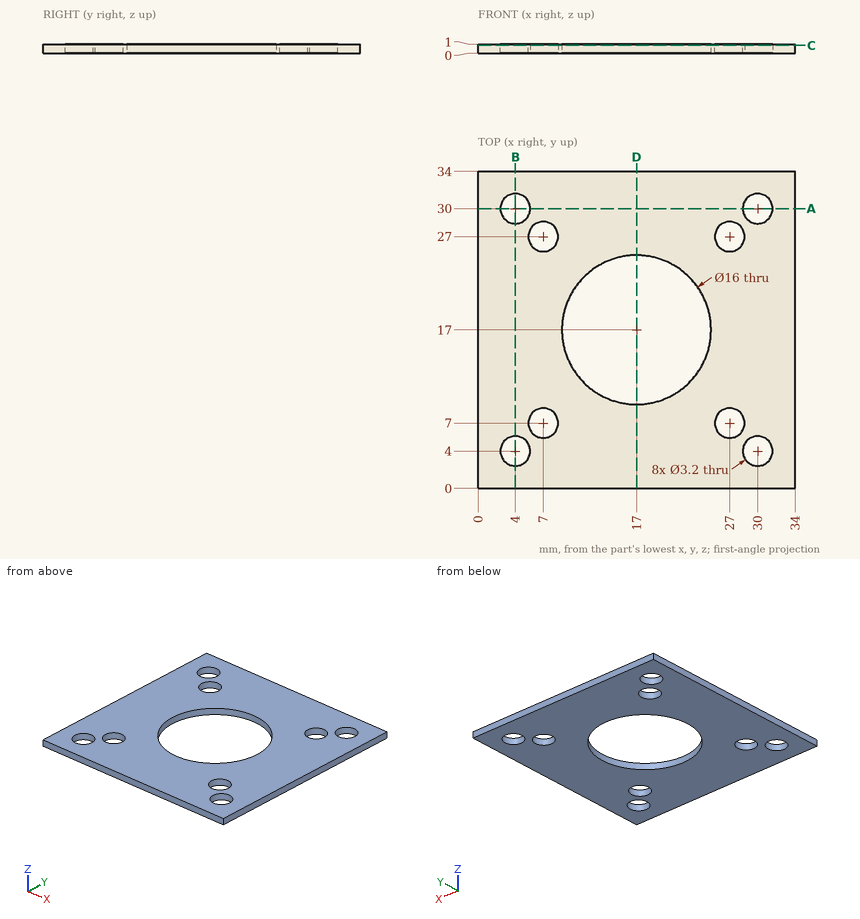
Check sheet for the drawn part. Datum: minimum x, y, z corner. Units: mm. Give positions to 0.01 mm unless a question says otherwise; leave off trailing zeros. Order: outer loops, then holes, each group sorted by start corner. A loop starts at its lowest first (then second) coordinate and runs counter-clockwise, first axis right, second up. Notation, with made-up numbers: (3.25, 30) -> (45.25, 30) arc R15 ccw to (45.25, 36) -> close; hole circle Ø9 at (18, 11.5). An arc over 180 degrees is marked (long way). Use a Markdown table: item, result.
1) Material ranges on probe 1 along Y at (x, z) = (27, 0.5); probe 2 along Y at (x, z) = (4, 0.7); probe 3 along Y at (x, z) = (17, 0.45), recorded low to high.
Results:
| item | result |
|---|---|
| probe 1 | 0 to 5.4, 8.6 to 25.4, 28.6 to 34 |
| probe 2 | 0 to 2.4, 5.6 to 28.4, 31.6 to 34 |
| probe 3 | 0 to 9, 25 to 34 |
2) Section check C-C, the plane z = 0.85. Give the number of separate pieces and of enclosed holes in the cut face, then the cut area to 3 significant figures.
Results:
| item | result |
|---|---|
| separate pieces | 1 |
| enclosed holes | 9 |
| area | 891 mm² |
3) Section check A-A, the plane y = 30. Record the boundary of the cut face in (x, z), then the cut area to 3 significant figures.
Results:
| item | result |
|---|---|
| outline | (0, 0) -> (2.4, 0) -> (2.4, 1) -> (0, 1) -> close; (5.6, 0) -> (28.4, 0) -> (28.4, 1) -> (5.6, 1) -> close; (31.6, 0) -> (34, 0) -> (34, 1) -> (31.6, 1) -> close |
| area | 27.6 mm² |
4) Section check D-D, the plane x = 17. Record the boundary of the cut face in (y, z).
Results:
| item | result |
|---|---|
| outline | (0, 0) -> (9, 0) -> (9, 1) -> (0, 1) -> close; (25, 0) -> (34, 0) -> (34, 1) -> (25, 1) -> close |
